Can you work these out from the model? Positions are in its coordinate system, mm. A direction names the side the tool comes from. Round coordinates to 2 decimals unless told otherwise and drop trailing zeros. Loops run counter-clockwise (first coordinate to the right, second up) from the corner with the lowest first, then second, coordinate; pieces in that order, holes last. Notation, with made-up numbers: (-0.75, -7) -> (38.25, -7) arc R19 ccw to (38.25, 10) -> close; hole circle Ø10 at (13.5, -33.5). An arc over 180 degrees is marked (long way). Write item = value, one per line.
from build123d import *

# Parameters (mm, degrees)
F0_W     = 86.36
F0_H     = 203.2
F1_DEPTH = 45.72
F3_DEPTH = 43.18
F5_DEPTH = 2.54
F6_W     = 82.3488
F6_H     = 42.672
F7_DEPTH = 2.286


with BuildPart() as f1:
    # F0 (on Front) → F1 (new body)
    with BuildSketch(Plane.XZ):
        with Locations((43.18, -101.6)):
            Rectangle(F0_W, F0_H)
    extrude(amount=-F1_DEPTH)

    # F2 (on face) → F3 (cut)
    with BuildSketch(Plane.XZ):
        Polygon((84.44604, -2.54), (2.097583, -2.302555), (2.097583, -48.022555), (84.44604, -48.26), align=None)
        Polygon((84.44604, -101.6), (84.44604, -55.88), (2.097583, -55.642555), (2.097583, -101.362555), align=None)
        Polygon((84.31421, -154.93981), (84.44604, -109.22), (2.097583, -108.982555), (2.097583, -154.702555), align=None)
    extrude(amount=-F3_DEPTH, mode=Mode.SUBTRACT)

    # F4 (on face) → F5 (join)
    with BuildSketch(Plane.XZ):
        Polygon((84.292239, -199.389778), (84.292239, -162.559778), (2.097583, -162.322555), (2.097583, -199.152555), align=None)
    extrude(amount=F5_DEPTH)

    # F6 (on face) → F7 (cut)
    with BuildSketch(Plane(origin=(-0.13845, 0, -48.016108), x_dir=(0.999996, 0, -0.002883), z_dir=(0.002883, 0, 0.999996))):
        with Locations((43.410442, 21.844)):
            Rectangle(F6_W, F6_H)
    extrude(amount=-F7_DEPTH, mode=Mode.SUBTRACT)


solid = f1.part
1. Suppose I cut it at D-D, the plane x = 81.5. List the corners of the cut face in (y, z) for me.
Entries:
outline = (-2.54, -199.38) -> (0, -199.38) -> (0, -203.2) -> (45.72, -203.2) -> (45.72, 0) -> (0, 0) -> (0, -2.53) -> (43.18, -2.53) -> (43.18, -50.54) -> (0.51, -50.54) -> (0.51, -48.25) -> (0, -48.25) -> (0, -55.87) -> (43.18, -55.87) -> (43.18, -101.59) -> (0, -101.59) -> (0, -109.21) -> (43.18, -109.21) -> (43.18, -154.93) -> (0, -154.93) -> (0, -162.55) -> (-2.54, -162.55) -> close
2. I need wall thicknesses on line 1 (Z direction, x = 18, y = 31); line 2 (Z direction, x = 81, y = 32.5); line 3 (X direction, y = 29, z = -84.5). Which ranges of each line are inside material? Lowest first, please. Write a range as [from, to].
Entries:
line_1 = [-203.2, -154.75], [-109.03, -101.41], [-55.69, -50.35], [-2.35, 0]
line_2 = [-203.2, -154.93], [-109.21, -101.59], [-55.87, -50.54], [-2.53, 0]
line_3 = [0, 2.1], [84.45, 86.36]
3. Suppose I cut it at C-C, the plane z = -32. List the corners of the cut face in (x, y) for me.
Entries:
outline = (0, 0) -> (2.1, 0) -> (2.1, 43.18) -> (84.45, 43.18) -> (84.45, 0) -> (86.36, 0) -> (86.36, 45.72) -> (0, 45.72) -> close
4. Suppose I cut it at A-A, the plane y = 6.5. List the corners of the cut face in (x, z) for me, and give its area (3 significant figures).
Entries:
outline = (0, -203.2) -> (86.36, -203.2) -> (86.36, 0) -> (0, 0) -> close; hole (2.09, -50.31) -> (84.44, -50.55) -> (84.45, -48.26) -> (84.45, -2.54) -> (2.1, -2.3) -> (2.1, -48.02) -> close; hole (2.1, -154.7) -> (84.31, -154.94) -> (84.45, -109.22) -> (2.1, -108.98) -> close; hole (2.1, -101.36) -> (84.45, -101.6) -> (84.45, -55.88) -> (2.1, -55.64) -> close
area = 6,070 mm²
5. Suppose I cut it at B-B, the plane x = 64. List the corners of the cut face in (y, z) for me.
Entries:
outline = (-2.54, -199.33) -> (0, -199.33) -> (0, -203.2) -> (45.72, -203.2) -> (45.72, 0) -> (0, 0) -> (0, -2.48) -> (43.18, -2.48) -> (43.18, -50.49) -> (0.51, -50.49) -> (0.51, -48.2) -> (0, -48.2) -> (0, -55.82) -> (43.18, -55.82) -> (43.18, -101.54) -> (0, -101.54) -> (0, -109.16) -> (43.18, -109.16) -> (43.18, -154.88) -> (0, -154.88) -> (0, -162.5) -> (-2.54, -162.5) -> close
6. I'm going to push flat-ended pins straight in: pin 1 (8 mm diameter, centred on x = 42.5, z = -67, fed in from -Y); pin 2 (1.3 mm diameter, centred on y = -1.5, z = -187, fed in from -X); pin 3 (12 mm diameter, centred on x = 74, z = -44, fed in from -Y). Where does each tip first touch, or does it pass through?
Entries:
pin_1 = 43.18
pin_2 = 2.1
pin_3 = 0
7. For faces 1 (the flat face through (43, 43.18, -132)), 2 (the flat face through (43, 23, -203.2)), which set-ups out of +Z, -Z, +X, -X, +Y, -Y let a thin tool reach every point of the face, with its end or its side?
Entries:
face_1 = -Y
face_2 = -Z, +X, -X, +Y, -Y
